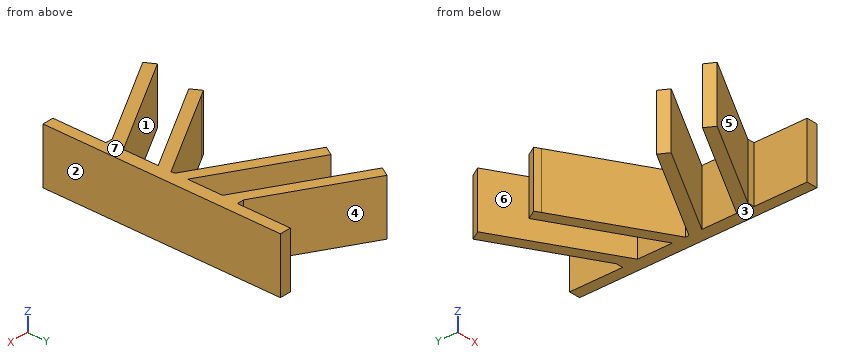
```python
from build123d import *

# Parameters (mm, degrees)
BOSS_EXTRUDE1_DEPTH = 8


with BuildPart() as part:
    # Sketch1 → Boss-Extrude1 (new body)
    with BuildSketch(Plane(origin=(0, 0, 0), x_dir=(0, 1, 0), z_dir=(0, 0, 1))):
        Polygon((-16.6, -1.8), (-16.6, -0.2), (-9, -0.2), (-9, 0.8), (-17.082903769, 14.8), (-15.697263123, 15.6), (-6.690598923, 0), (-1.690598923, 0), (-9.773502692, 14), (-8.387862046, 14.8), (-7.935720847, 14.016868471), (0.172032948, -0.026173037), (0.672032948, -0.026173037), (8.779786743, 14.016868471), (9.231927942, 14.8), (10.617568588, 14), (2.534664819, 0), (7.534664819, 0), (16.541329018, 15.6), (17.926969664, 14.8), (9.844065896, 0.8), (9.844065896, -0.2), (17.444065896, -0.2), (17.444065896, -1.8), (0.422032948, -1.8), align=None)
    extrude(amount=BOSS_EXTRUDE1_DEPTH)


solid = part.part
```
For this review, take the finished solid that the model builds, in its own axes (mm). Face numbers are marked on the shaded views. A direction names the side the tool comes from. Round coordinates to 2 decimals unless told otherwise and drop trailing zeros. Write each loop counter-clockwise with the first axis right and the second up, starting at its lowest first coordinate (ties: lowest second). Pieces come first, ordered by that corner, then holes. Notation, with made-up numbers: (73, 15.5) - (113, 15.5) arc R30 cw to (113, 40.5) - close; hole circle Ø3 at (-16, 72). An arc over 180 degrees is marked (long way). Answer as CSV lines item,"result". Start each with the question number.
(1) Add section B-B, the plane x = -9. State the section outline as (y, z) points.
(2) For pin 1 (1.3 mm diameter, centred on x = 1, z = 6, fed in from +Y); pin 2 (2.5 mm diameter, centred on y = 5, z = 4.5, fed in from -X); pin 3 (2 mm diameter, centred on y = -9, z = 7, fed in from -X), all flat-tipped, find the tip position at first contact; note any pin that passes through.
(3) Add section C-C, the plane z = 5. State the section outline as (x, y) points, plus the area to 3 significant figures.
(4) Machinability: for the marked faces 4, 5, 6 and 7, which of the approach directions +Z, -Z, +X, -X, +Y, -Y give a long, thin tool a straight path to every point of the face, cutting with its end or side? Answer none if there is none.
(5) Add section A-A, the plane y = 15. State the section outline as (x, z) points.
(6) Add section D-D, the plane y = -4.5. State the section outline as (x, z) points, plus the area to 3 significant figures.
(7) Mouldability with a two-part tool opening along X and no side actions: class the marked faces 1, 2 and 3 as +X half, -X half, draft (parallel to the pull), parting line (faces both ways), or undercut.
(8) For line 1 (Y direction, x = -9.75, z = 1.25); line 2 (Y direction, x = -3.5, z = 2.5); line 3 (X direction, y = -11, z = 1), list the stretches that pass through material, from the lowest coordinate up.
From the geometry:
1,outline,"(-13.73, 0) - (-11.89, 0) - (-11.89, 8) - (-13.73, 8) - close; (-6.89, 0) - (-5.04, 0) - (-5.04, 8) - (-6.89, 8) - close; (5.88, 0) - (7.73, 0) - (7.73, 8) - (5.88, 8) - close; (12.73, 0) - (14.58, 0) - (14.58, 8) - (12.73, 8) - close"
2,pin 1,"stops at y = 17.44"
2,pin 2,"stops at x = -9.64"
2,pin 3,"stops at x = -14.8"
3,outline,"(-15.6, -15.7) - (-14.8, -17.08) - (-0.8, -9) - (0.2, -9) - (0.2, -16.6) - (1.8, -16.6) - (1.8, 17.44) - (0.2, 17.44) - (0.2, 9.84) - (-0.8, 9.84) - (-14.8, 17.93) - (-15.6, 16.54) - (0, 7.53) - (0, 2.53) - (-14, 10.62) - (-14.8, 9.23) - (0.03, 0.67) - (0.03, 0.17) - (-14.8, -8.39) - (-14, -9.77) - (0, -1.69) - (0, -6.69) - close"
3,area,"168 mm²"
4,face 4,"+Z, -Z, +Y"
4,face 5,"+Z, -Z, -Y"
4,face 6,"+Z, -Z"
4,face 7,"+Z, +X, -X, +Y, -Y"
5,outline,"(-12.93, 0) - (-9.73, 0) - (-9.73, 8) - (-12.93, 8) - close; (0.2, 0) - (1.8, 0) - (1.8, 8) - (0.2, 8) - close"
6,outline,"(-8.07, 0) - (-4.87, 0) - (-4.87, 8) - (-8.07, 8) - close; (0, 0) - (1.8, 0) - (1.8, 8) - (0, 8) - close"
6,area,"40.0 mm²"
7,face 1,"undercut"
7,face 2,"+X half"
7,face 3,"draft"
8,line 1,"y = -14.17 to -12.32, -7.32 to -5.47, 6.32 to 8.16, 13.16 to 15.01"
8,line 2,"y = -10.56 to -8.71, -3.71 to -1.86, 2.71 to 4.56, 9.56 to 11.4"
8,line 3,"x = -7.46 to -4.26, 0.2 to 1.8"
